Geometry: see drawing. Coordinates: mm, zero at the bounding-box minimum. Give positions to 0.01 mm unless a question says otherwise; leave off trailing zeros. Order: outer loops, then holes, each group sorted by start corner. A loop starts at its lowest first (then second) coordinate and runs counter-clockwise, first axis right, second up. Notation, with made-up numbers: (62.25, 84.25) - (85.25, 84.25) arc R18 cw to (85.25, 108.25) - close; hole circle Ø4 at (82.25, 57). An arc over 180 degrees is marked (long way). One line per item, written item: value. Start each with the question number.
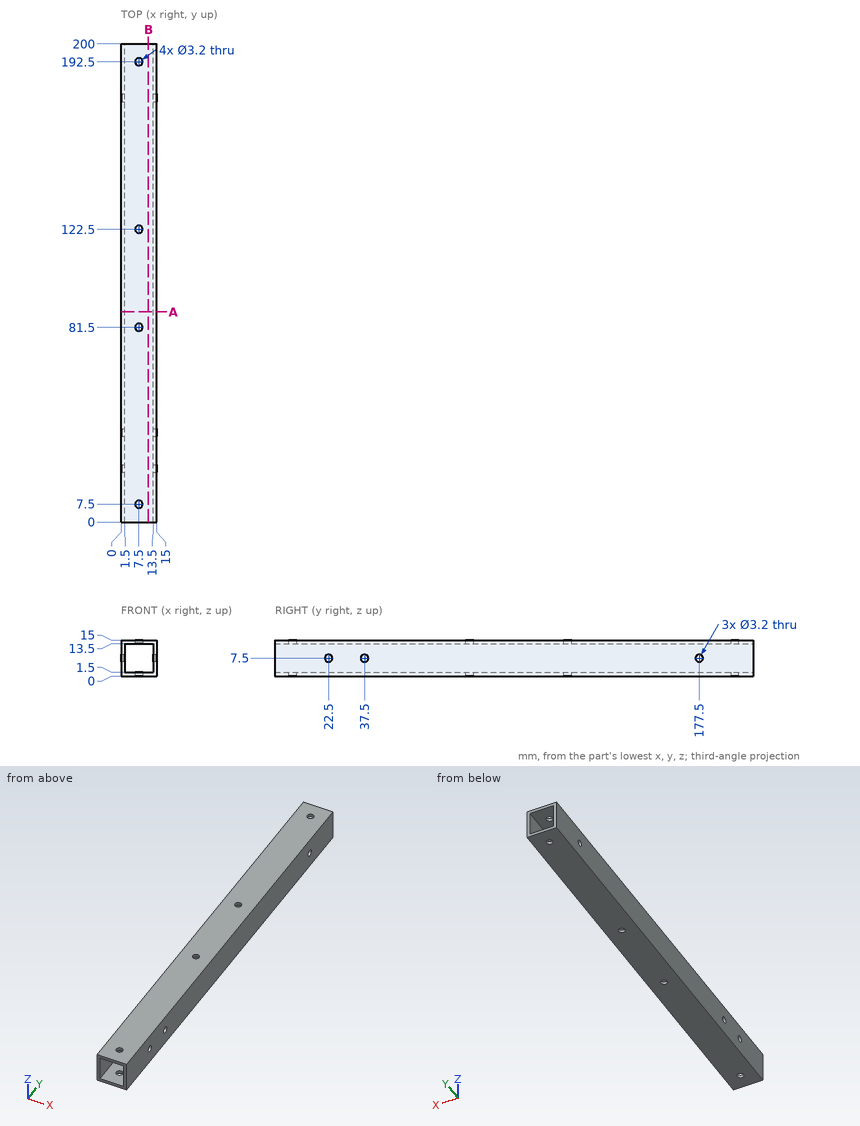
1. Section A-A on y = 88. Return the cut outline in (x, z).
2. Ray query, L1, parallel to Y at x = 0.85, z = 7.5; L2, parallel to Z at x = 6.25, y = 177.5; L3, parallel to X at y = 192.5, z = 14.6. Return the intervals inside material, ascending.
3. Section B-B on x = 11.5. Return the cut outline in (y, z).
Data:
1. outline: (0, 0) - (15, 0) - (15, 15) - (0, 15) - close; hole (1.5, 1.5) - (13.5, 1.5) - (13.5, 13.5) - (1.5, 13.5) - close
2. L1: y = 0 to 20.9, 24.1 to 35.9, 39.1 to 175.9, 179.1 to 200
2. L2: z = 0 to 1.5, 13.5 to 15
2. L3: x = 0 to 5.9, 9.1 to 15
3. outline: (0, 0) - (200, 0) - (200, 1.5) - (0, 1.5) - close; (0, 13.5) - (200, 13.5) - (200, 15) - (0, 15) - close
